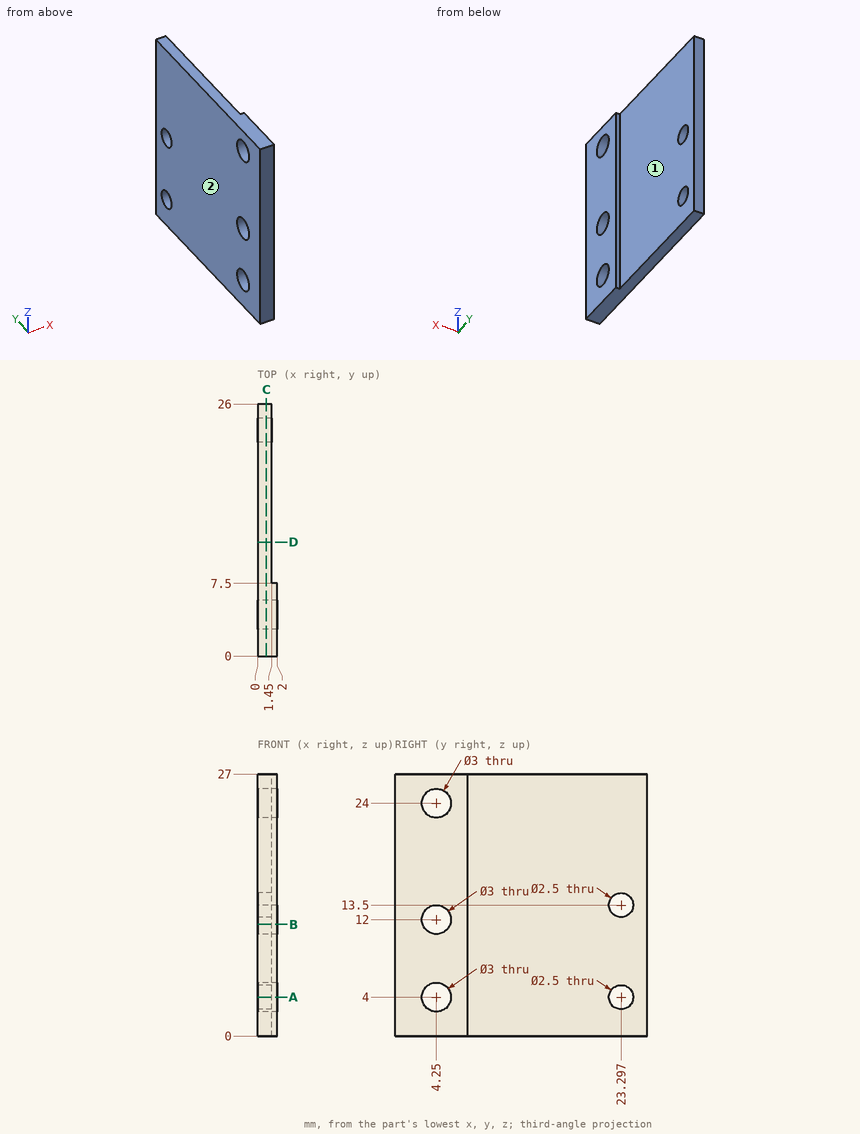
Verification items for this drawing (mm, ordinates from the low corner). A direction names the side the tool comes from. Give positions to 0.01 mm unless a question says otherwise; leave off trailing zeros. Loops run counter-clockwise (first coordinate to the right, second up) from the corner with the lowest first, then second, coordinate; pieces in that order, holes last. Notation, with made-up numbers: M 33,-26.5 L 57,-26.5 A24 ccw 57,12.5 Z; hole C -38.5,-24 d11. An arc over 180 degrees is marked long. Answer in a Markdown table with one row per item.
1) Cross-section at C-C (x = 0.9). Enter the section's corners in (y, z).
Solutions:
| item | result |
|---|---|
| outline | M 0,0 L 26,0 L 26,27 L 0,27 Z; hole C 4.25,4 d3; hole C 4.25,12 d3; hole C 4.25,24 d3; hole C 23.3,4 d2.5; hole C 23.3,13.5 d2.5 |
2) Cross-section at A-A (z = 4). Enter the section's corners in (x, y), plus the area to 3 significant figures.
Solutions:
| item | result |
|---|---|
| outline | M 0,0 L 2,0 L 2,2.75 L 0,2.75 Z; M 0,5.75 L 2,5.75 L 2,7.5 L 1.45,7.5 L 1.45,22.05 L 0,22.05 Z; M 0,24.55 L 1.45,24.55 L 1.45,26 L 0,26 Z |
| area | 32.2 mm^2 |
3) Cross-section at B-B (z = 11.5). Enter the section's corners in (x, y).
Solutions:
| item | result |
|---|---|
| outline | M 0,0 L 2,0 L 2,2.84 L 0,2.84 Z; M 0,5.66 L 2,5.66 L 2,7.5 L 1.45,7.5 L 1.45,26 L 0,26 Z |
4) Depth check by flat-ended pin: pin 1 (2.5 mm diameter, centred on y = 4.25, z = 4, fed in from +X); pin 2 (9 mm diameter, centred on y = 17, z = 17.5, fed in from +X); pin 3 (0.6 mm diameter, centred on x = 2, z = 7.5, fed in from +Y). Enter the tip coordinate at first touch or a pass-through.
Solutions:
| item | result |
|---|---|
| pin 1 | passes through |
| pin 2 | stops at x = 1.45 |
| pin 3 | stops at y = 7.5 |
5) Thickness scan on line 1 (Y direction, x = 1.1, z = 4); line 2 (Y direction, x = 0.7, z = 12); line 3 (Z direction, x = 0.7, y = 23.5). Record the ranges inside material, lowest first.
Solutions:
| item | result |
|---|---|
| line 1 | y = 0 to 2.75, 5.75 to 22.05, 24.55 to 26 |
| line 2 | y = 0 to 2.75, 5.75 to 26 |
| line 3 | z = 0 to 2.77, 5.23 to 12.27, 14.73 to 27 |
6) Cross-section at D-D (y = 11.75). Enter the section's corners in (x, z).
Solutions:
| item | result |
|---|---|
| outline | M 0,0 L 1.45,0 L 1.45,27 L 0,27 Z |
7) Tool access check on the marked faces 1 and 2. Record the directions out of +Z, -Z, +X, -X, +Y, -Y that give a thin tool (end or side, any length) a straight path to the whole face; none if there is none.
Solutions:
| item | result |
|---|---|
| face 1 | +Z, -Z, +X, +Y |
| face 2 | +Z, -Z, -X, +Y, -Y |
